```python
from build123d import *

# Parameters (mm, degrees)
SKETCH2_W           = 44
SKETCH2_H           = 200
BOSS_EXTRUDE2_DEPTH = 8.5
SKETCH4_R           = 11.04
CUT_EXTRUDE1_DEPTH  = 7.5
SKETCH5_OUTSIDE_W   = 86.992
SKETCH5_OUTSIDE_H   = 242.992
SKETCH5_OUTSIDE_R   = 8
CUT_EXTRUDE2_DEPTH  = 10
SKETCH6_R           = 14
BOSS_EXTRUDE3_DEPTH = 16.51
SKETCH8_R           = 6.096
CUT_EXTRUDE4_DEPTH  = 16.51


with BuildPart() as part:
    # Sketch2 → Boss-Extrude2 (new body)
    with BuildSketch(Plane(origin=(0, 0, 0), x_dir=(0, 0, -1), z_dir=(1, 0, 0))):
        with Locations((22, 100)):
            Rectangle(SKETCH2_W, SKETCH2_H)
    extrude(amount=BOSS_EXTRUDE2_DEPTH)

    # Sketch4 → Cut-Extrude1 (cut)
    with BuildSketch(Plane(origin=(0, 0, 0), x_dir=(0, 0, -1), z_dir=(1, 0, 0))):
        with Locations(Location((22, 22, 0), (0, 0, 180))):
            Circle(SKETCH4_R)
    extrude(amount=CUT_EXTRUDE1_DEPTH, mode=Mode.SUBTRACT)

    # Sketch5 outside → Cut-Extrude2 (cut)
    # profile 1 of 2: a face of its own
    with BuildSketch(Plane(origin=(8.5, 0, 0), x_dir=(0, 0, -1), z_dir=(1, 0, 0))):
        with Locations((22, 100)):
            Rectangle(SKETCH5_OUTSIDE_W, SKETCH5_OUTSIDE_H)
        with BuildLine():
            Line((11, 200), (11, 46.145392935))
            ThreePointArc((11, 46.145392935), (10.100137362, 41.999611947), (7.5625, 38.599957643))
            ThreePointArc((7.5625, 38.599957643), (22, 0), (36.4375, 38.599957643))
            ThreePointArc((36.4375, 38.599957643), (33.899862638, 41.999611947), (33, 46.145392935))
            Line((33, 46.145392935), (33, 200))
            Line((33, 200), (11, 200))
        make_face(mode=Mode.SUBTRACT)
    # profile 2 of 2: a face of its own
    with BuildSketch(Plane(origin=(8.5, 0, 0), x_dir=(0, 0, -1), z_dir=(1, 0, 0))):
        with Locations((22, 22)):
            Circle(SKETCH5_OUTSIDE_R)
    extrude(amount=-CUT_EXTRUDE2_DEPTH, mode=Mode.SUBTRACT)

    # Sketch6 → Boss-Extrude3 (add)
    with BuildSketch(Plane(origin=(8.5, 0, 0), x_dir=(0, 0, -1), z_dir=(1, 0, 0))):
        with Locations(Location((22, 22, 0), (0, 0, 180))):
            Circle(SKETCH6_R)
    extrude(amount=BOSS_EXTRUDE3_DEPTH)

    # Sketch8 → Cut-Extrude4 (cut)
    with BuildSketch(Plane(origin=(25.01, 0, 0), x_dir=(0, 0, -1), z_dir=(1, 0, 0))):
        with Locations((22, 22)):
            Circle(SKETCH8_R)
    extrude(amount=-CUT_EXTRUDE4_DEPTH, mode=Mode.SUBTRACT)


solid = part.part
```
Model file for the job. Use its own axes, mm. A direction names the side the tool comes from. Coordinates: 2 decimals unless noted, no trailing zeros. Write each loop counter-clockwise with the first axis right and the second up, starting at its lowest first coordinate (ties: lowest second). Pieces come first, ordered by that corner, then holes. Notation, with made-up numbers: (-11.75, -28) - (24.25, -28) arc R4 ccw to (24.25, -24) - close; hole circle Ø5 at (69.5, 74). An arc over 180 degrees is marked (long way). Use a Markdown table: item, result. Add a question column.
Item 1: Band-saw the part on D-D, the plane y = 126. Write the cut outline in (x, z).
Item 2: Drop flat-ended pins along their axis: pin 1 (13 mm diameter, centred on y = 71, z = -24.5, fed in from +X); pin 2 (4 mm diameter, centred on x = 9, y = 46.5, fed in from -Z); pin 3 (17.5 mm diameter, centred on y = 25.5, z = -24, fed in from -X); pin 4 (9.5 mm diameter, centred on x = 6, y = 144, fed in from -Z). Give the stop position or say it passes through.
Item 3: 3-axis set-ups, long thin cutter, end or side, ignore diameter. For faces 1 (the face through (8, 27.4, -16.1)), 2 (the face through (25.01, 28, -19)), 3 (the face through (16.64, 35.67, -25.03)): which of +Z, -Z, +X, -X, +Y, -Y reach the whole face in a straight line?
Item 4: Two-plate mould, pull along Z, no slides. Class faces 4 (the face through (4, 122, -33)), 5 (the face through (4, 124, -11)), 6 (the face through (16.87, 16.05, -20.68)), 7 (the face through (3.698, 12.691, -16.065)): pulls with the +Z half, pulls with the -Z half, needs draft (parallel to the pull), parting line crosses it, or undercut.
Item 5: Drill centre lines: line 1 along Y through (x, z) = (8.05, -22); line 2 along Z through (x, y) = (3.5, 22); line 3 along Y through (x, z) = (5, -22). Where is each one in solid material? Low to high.
Item 6: Band-saw the part on C-C, the plane z = -18. Write the cut outline in (x, y).
Item 7: Band-saw the part on A-A, the plane y = 22. Write the cut outline in (x, z), and give its area (3 significant figures).
Item 8: Band-saw the part on B-B, the plane x = 5. Write the cut outline in (y, z), and give its area (3 significant figures).
A:
| question | item | result |
|---|---|---|
| 1 | outline | (0, -33) - (8.5, -33) - (8.5, -11) - (0, -11) - close |
| 2 | pin 1 | stops at x = 8.5 |
| 2 | pin 2 | stops at z = -33.13 |
| 2 | pin 3 | stops at x = 0 |
| 2 | pin 4 | stops at z = -33 |
| 3 | face 1 | -X |
| 3 | face 2 | +Z, -Z, +X, +Y, -Y |
| 3 | face 3 | +X |
| 4 | face 4 | pulls with the -Z half |
| 4 | face 5 | pulls with the +Z half |
| 4 | face 6 | undercut |
| 4 | face 7 | undercut |
| 5 | line 1 | y = 0 to 14, 30 to 200 |
| 5 | line 2 | z = -44 to -33.04, -10.96 to 0 |
| 5 | line 3 | y = 0 to 10.96, 33.04 to 200 |
| 6 | outline | (0, 0.37) - (8.5, 0.37) - (8.5, 8.58) - (25.01, 8.58) - (25.01, 17.4) - (8.5, 17.4) - (8.5, 15.07) - (7.5, 15.07) - (7.5, 11.71) - (0, 11.71) - close; (0, 32.29) - (7.5, 32.29) - (7.5, 28.93) - (8.5, 28.93) - (8.5, 26.6) - (25.01, 26.6) - (25.01, 35.42) - (8.5, 35.42) - (8.5, 200) - (0, 200) - close |
| 7 | outline | (0, -44) - (8.5, -44) - (8.5, -36) - (25.01, -36) - (25.01, -28.1) - (8.5, -28.1) - (8.5, -30) - (7.5, -30) - (7.5, -33.04) - (0, -33.04) - close; (0, -10.96) - (7.5, -10.96) - (7.5, -14) - (8.5, -14) - (8.5, -15.9) - (25.01, -15.9) - (25.01, -8) - (8.5, -8) - (8.5, 0) - (0, 0) - close |
| 7 | area | 453 mm² |
| 8 | outline | (38.6, -36.44) arc R10 cw to (46.15, -33) - (200, -33) - (200, -11) - (46.15, -11) arc R10 cw to (38.6, -7.56) arc R22 ccw (long way) to start; hole circle Ø22.08 at (22, -22) |
| 8 | area | 4,600 mm² |
